Verification items for the finished model (mm, model axes). A direction names the side the tool comes from. Coordinates: 2 decimals unless noted, no trailing zeros. Order: outer loops, then holes, each group sorted by start corner. A loop starts at its lowest first (then second) coordinate and runs counter-clockwise, first axis right, second up.
Q1. Cross-section at C-C, the plane z = -7. Record the boundary of the cut face in (x, y).
Q2. Cross-section at A-A, the plane y = -18.5. Record the boundary of the cut face in (x, z).
Q3. Set-up check for faces 5 (the flat face through (-26, -25, 9.887)), 6 (the flat face through (-1, -25, -8.15)), 7 (the cylindrical face through (-9.74, -20.34, 6.02)): record each of +Z, -Z, +X, -X, +Y, -Y from which the full face is reachable in a straight line by a thin tool's end or side.
Q4. Thickness scan on line 1 (Z direction, x = -1.5, y = -19.5); line 2 (Z direction, x = -5, y = -16); line 3 (X direction, y = -23, z = -44). Record the ranges inside material, lowest first.
Q5. Cross-section at B-B, the plane x = -6. Record the boundary of the cut face in (y, z).
Q6. Draft check along Z on faces 1 (the flat face through (5, -25, -28.233)), 2 (the flat face through (-26, -25, -58.733)), 3 (the flat face through (-26, -50.8, -25)), 4 (the flat face through (-12, -24, 2.267)). Enter one of: pulls with the +Z half, pulls with the -Z half, needs draft (parallel to the pull), parting line crosses it, or undercut.
Q7. Cross-section at D-D, the plane y = -26. Record the boundary of the cut face in (x, z), and give its area (3 significant figures).
Q8. Depth check by flat-ended pin: P1, Ø15, axis at x = -7.03, z = -36.14, coming from the +Y side; P2, Ø4.5, axis at x = -11.83, y = -23.62, coming from the +Z side; P3, Ø0.8, axis at y = -28, z = -7.5, coming from the +X side. Enter the tip coordinate at first touch or a pass-through.
from build123d import *

# Parameters (mm, degrees)
F1_DEPTH = 50.8
F2_W     = 67
F2_H     = 50.8
F2_R     = 3.887383
F3_DEPTH = 7.62


with BuildPart() as f1:
    # F0 (on Front) → F1 (new body)
    with BuildSketch(Plane.XZ):
        with BuildLine():
            Line((8.097237, 2.266741), (-58.902763, 2.266741))
            Line((-58.902763, 2.266741), (-58.902763, -58.733259))
            Line((-58.902763, -58.733259), (8.097237, -58.733259))
            Line((8.097237, -58.733259), (8.097237, -37.91259))
            Line((8.097237, -37.91259), (5.399642, -37.91259))
            ThreePointArc((5.399642, -37.91259), (-19.132664, -39.489125), (2.721969, -28.233259))
            Line((2.721969, -28.233259), (8.097237, -28.233259))
            Line((8.097237, -28.233259), (8.097237, -8.149563))
            Line((8.097237, -8.149563), (-9.469079, -8.149563))
            Line((-9.469079, -8.149563), (-9.469079, -5.638948))
            Line((-9.469079, -5.638948), (8.097237, -5.638948))
            Line((8.097237, -5.638948), (8.097237, 2.266741))
        make_face()
    extrude(amount=F1_DEPTH)

    # F2 (on face) → F3 (join)
    with BuildSketch(Plane.XY.offset(2.266741)):
        with Locations((-25.402763, -25.4)):
            Rectangle(F2_W, F2_H)
        with Locations((-11.831898, -23.617744)):
            Circle(F2_R, mode=Mode.SUBTRACT)
    extrude(amount=F3_DEPTH)


solid = f1.part
Check values:
1. outline: (-58.9, -50.8) - (-9.47, -50.8) - (-9.47, 0) - (-58.9, 0) - close
2. outline: (-58.9, -58.73) - (8.1, -58.73) - (8.1, -37.91) - (5.4, -37.91) arc R12.56 cw (long way) to (2.72, -28.23) - (8.1, -28.23) - (8.1, -8.15) - (-9.47, -8.15) - (-9.47, -5.64) - (8.1, -5.64) - (8.1, 9.89) - (-58.9, 9.89) - close
3. face 5: +Z, +X, -X, +Y, -Y
3. face 6: +X, +Y, -Y
3. face 7: +Z
4. line 1: z = -58.73 to -47.41, -24.87 to -8.15, -5.64 to 9.89
4. line 2: z = -58.73 to -48.53, -23.75 to -8.15, -5.64 to 9.89
4. line 3: x = -58.9 to -16.82, 2.76 to 8.1
5. outline: (-50.8, -58.73) - (0, -58.73) - (0, -48.66) - (-50.8, -48.66) - close; (-50.8, -23.63) - (0, -23.63) - (0, -8.15) - (-50.8, -8.15) - close; (-50.8, -5.64) - (0, -5.64) - (0, 9.89) - (-50.8, 9.89) - close
6. face 1: undercut
6. face 2: pulls with the -Z half
6. face 3: needs draft
6. face 4: pulls with the +Z half
7. outline: (-58.9, -58.73) - (8.1, -58.73) - (8.1, -37.91) - (5.4, -37.91) arc R12.56 cw (long way) to (2.72, -28.23) - (8.1, -28.23) - (8.1, -8.15) - (-9.47, -8.15) - (-9.47, -5.64) - (8.1, -5.64) - (8.1, 9.89) - (-8.76, 9.89) - (-8.76, 2.27) - (-14.9, 2.27) - (-14.9, 9.89) - (-58.9, 9.89) - close
7. area: 3,980 mm2
8. P1: passes through
8. P2: stops at z = 2.27
8. P3: stops at x = -9.47
